Geometry check sheet. Reference: the model listing, model coordinates, mm. Give positions to 0.01 mm unless a question says otherwise; leave off trailing zeros. Loops run counter-clockwise (first coordinate to the right, second up) from the corner with the lowest first, then second, coordinate; pieces in that order, holes last. Notation, with made-up numbers: (20, 1.5) -> (35, 1.5) arc R13 ccw to (35, 10.5) -> close; hole circle Ø10 at (73, 79). An arc over 180 degrees is marked (long way). Write each question's results on one line, items separated by ' | '. Start each with the question number.
1) Scan lines: line 1 (Z direction, x = -32, y = -8); line 2 (X direction, y = -1.5, z = 20.5); line 3 (X direction, y = -8, z = 7). Record each from-to range of solid material in increasing order. Write a range as from..to.
2) Draft check along X on faces 1 (the face through (28.58, 0.14, 6.44)), 2 (the face through (3.441, 15.497, 19.139)), 3 (the face through (16, -1, 12.7)). Enter one of: pulls with the +X half, pulls with the -X half, needs draft (parallel to the pull), parting line crosses it, or undercut.
3) Sectioned sample at C-C on z = 16. Record the cut outline in (x, y) (3 decimals), then the cut area to 3 significant figures.
4) Sectioned sample at D-D on z = 8. Record the cut outline in (x, y) (3 decimals).
5) Depth check by flat-ended pin: pin 1 (10 mm diameter, centred on x = -31.75, y = 0, fed in from +Z); pin 2 (3 mm diameter, centred on y = 12, z = 6, fed in from -X); pin 3 (4 mm diameter, centred on x = 0, y = -31.75, fed in from +Z); pin 4 (6 mm diameter, centred on x = -14, z = 22, fed in from +Y). Enter the tip coordinate at first touch or a pass-through.
6) Sectioned sample at A-A on x = 0. Record the cut outline in (y, z) (3 decimals), then the cut area to 3 significant figures.
```python
from build123d import *

# Parameters (mm, degrees)
F0_W     = 15.875
F0_H     = 12.7
F2_R     = 3.175
F3_DEPTH = 25.4
F4_R     = 9.525
F5_DEPTH = 50.5226


with BuildPart() as f1:
    # F0 (on Front) → F1 (revolve)
    with BuildSketch(Plane.XZ):
        Polygon((-38.1, 0), (0, 0), (0, 12.7), (-15.875, 12.7), (-38.1, 12.7), align=None)
        with Locations((-7.9375, 19.05)):
            Rectangle(F0_W, F0_H)
    revolve(axis=Axis((0, 0, 18.219382), (0, 0, 1)))

    # F2 (on face) → F3 (cut)
    with BuildSketch(Plane.XY.offset(12.7)):
        with Locations((0, 31.75)):
            Circle(F2_R)
        with Locations((-31.75, 0)):
            Circle(F2_R)
        with Locations((0, -31.75)):
            Circle(F2_R)
        with Locations((31.75, 0)):
            Circle(F2_R)
    extrude(amount=-F3_DEPTH, mode=Mode.SUBTRACT)

    # F4 (on face) → F5 (cut)
    with BuildSketch(Plane.XY.offset(25.4)):
        Circle(F4_R)
    extrude(amount=-F5_DEPTH, mode=Mode.SUBTRACT)


solid = f1.part
```
Result:
1) line 1: 0..12.7 | line 2: -15.8..-9.41, 9.41..15.8 | line 3: -37.25..-5.17, 5.17..37.25
2) face 1: undercut | face 2: parting line crosses it | face 3: needs draft
3) outline: circle Ø31.75 at (0, 0); hole circle Ø19.05 at (0, 0) | area: 507 mm^2
4) outline: circle Ø76.2 at (0, 0); hole circle Ø6.35 at (-31.75, 0); hole circle Ø19.05 at (0, 0); hole circle Ø6.35 at (0, -31.75); hole circle Ø6.35 at (0, 31.75); hole circle Ø6.35 at (31.75, 0)
5) pin 1: z = 12.7 | pin 2: x = -36.62 | pin 3: through | pin 4: y = 11.45
6) outline: (-38.1, 0) -> (-34.925, 0) -> (-34.925, 12.7) -> (-38.1, 12.7) -> close; (-28.575, 0) -> (-9.525, 0) -> (-9.525, 25.4) -> (-15.875, 25.4) -> (-15.875, 12.7) -> (-28.575, 12.7) -> close; (9.525, 0) -> (28.575, 0) -> (28.575, 12.7) -> (15.875, 12.7) -> (15.875, 25.4) -> (9.525, 25.4) -> close; (34.925, 0) -> (38.1, 0) -> (38.1, 12.7) -> (34.925, 12.7) -> close | area: 726 mm^2
